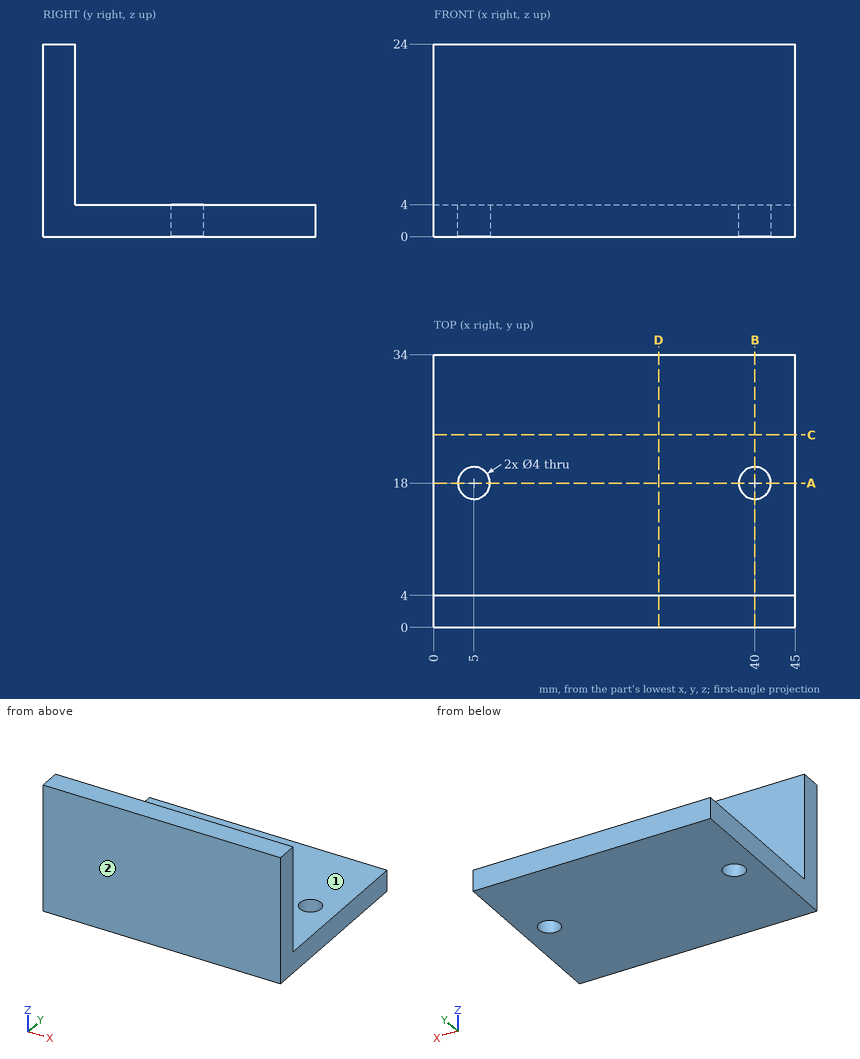
Check sheet for the drawn part. Datum: minimum x, y, z corner. Units: mm. A direction names the side the tool comes from. Give positions to 0.01 mm unless a question says otherwise; leave off trailing zeros. Order: outer loops, then holes, each group sorted by start corner. A loop starts at its lowest first (then second) coordinate and runs counter-clockwise, first axis right, second up. Notation, with made-up numbers: (-8.5, -1) -> (39.5, -1) arc R6 cw to (39.5, 4) -> close; hole circle Ø9 at (45, -8.5). An arc over 180 degrees is marked (long way). Use a Markdown table: item, result.
1) Section check A-A, the plane y = 18. Record the boundary of the cut face in (x, z), then the cut area to 3 significant figures.
Results:
| item | result |
|---|---|
| outline | (0, 0) -> (3, 0) -> (3, 4) -> (0, 4) -> close; (7, 0) -> (38, 0) -> (38, 4) -> (7, 4) -> close; (42, 0) -> (45, 0) -> (45, 4) -> (42, 4) -> close |
| area | 148 mm² |
2) Material ranges on probe 1 along Y at (x, z) = (40, 1.15); probe 2 along Z at (x, y) = (40, 14.5), recorded low to high.
Results:
| item | result |
|---|---|
| probe 1 | 0 to 16, 20 to 34 |
| probe 2 | 0 to 4 |
3) Section check B-B, the plane x = 40. Record the boundary of the cut face in (y, z).
Results:
| item | result |
|---|---|
| outline | (0, 0) -> (16, 0) -> (16, 4) -> (4, 4) -> (4, 24) -> (0, 24) -> close; (20, 0) -> (34, 0) -> (34, 4) -> (20, 4) -> close |
4) Tool access check on the marked faces 1 and 2. Record the directions out of +Z, -Z, +X, -X, +Y, -Y that give a thin tool (end or side, any length) a straight path to the whole face; none if there is none.
Results:
| item | result |
|---|---|
| face 1 | +Z, +X, -X, +Y |
| face 2 | +Z, -Z, +X, -X, -Y |
5) Section check D-D, the plane x = 28. Record the boundary of the cut face in (y, z).
Results:
| item | result |
|---|---|
| outline | (0, 0) -> (34, 0) -> (34, 4) -> (4, 4) -> (4, 24) -> (0, 24) -> close |
6) Depth check by flat-ended pin: pin 1 Ø5 at (x, y) = (8.5, 17) entering from +Z; pin 2 Ø1 at (x, z) = (5, 17) entering from +Y. Enter the tip coordinate at first touch or a pass-through.
Results:
| item | result |
|---|---|
| pin 1 | z = 4 |
| pin 2 | y = 4 |
7) Section check C-C, the plane y = 24. Record the boundary of the cut face in (x, z), then the cut area to 3 significant figures.
Results:
| item | result |
|---|---|
| outline | (0, 0) -> (45, 0) -> (45, 4) -> (0, 4) -> close |
| area | 180 mm² |
